Work out the finished part from the listing and answer in its coordinate system (mm). A direction names the side the tool comes from. Round coordinates to 2 decimals unless told otherwise and drop trailing zeros. Loops run counter-clockwise (first coordinate to the right, second up) from the corner with the lowest first, then second, coordinate; pieces in that order, holes last.
```python
from build123d import *

# Parameters (mm, degrees)
F0_W      = 76.2
F0_H      = 38.1
F1_DEPTH  = 25.4
F2_R      = 6.35
F1_FACE_W = 76.2
F1_FACE_H = 38.1
F3_DEPTH  = 25.4
F4_SIZE   = 2.53999
F5_R      = 10.16
F6_DEPTH  = 38.1
F7_R      = 5.08
F8_DEPTH  = 6.35
F9_R      = 10.16
F10_DEPTH = 6.35
F11_R     = 1.905
F12_DEPTH = 25.4
F13_DEPTH = 15.24
F14_R     = 2.54
F15_R     = 2.54
F16_R     = 2.54
F17_DEPTH = 50.8
F18_SIZE  = 3.81
F19_R     = 5.07999


# Not quite as in the source:
# - a fillet or chamfer is up to 0.001 mm smaller than in the source, because OpenCascade refuses the exact size


with BuildPart() as f1:
    # F0 (on Top) → F1 (new body)
    with BuildSketch(Plane.XY):
        with Locations((-5.318582058, 0.8709464072)):
            Rectangle(F0_W, F0_H)
    extrude(amount=F1_DEPTH)

    # F2 (on Top) + F1_face (on face) → F3 (cut)
    with BuildSketch(Plane.XY):
        with Locations((-34.528582058, -9.2890535928)):
            Circle(F2_R)
        with Locations((23.891417942, 11.0309464072)):
            Circle(F2_R)
        with Locations((23.891417942, -9.2890535928)):
            Circle(F2_R)
        with Locations((-34.528582058, 11.0309464072)):
            Circle(F2_R)
    with BuildSketch(Plane(origin=(-5.318582058, 0.8709464072, 25.4), x_dir=(1, 0, 0), z_dir=(0, 0, 1))):
        Rectangle(F1_FACE_W, F1_FACE_H)
    extrude(amount=F3_DEPTH, mode=Mode.SUBTRACT)

    # F4 (size 2.54 in the source; OpenCascade refuses exactly that, so slightly less here)
    f4_edges = [f1.edges().sort_by_distance(p)[0] for p in [
        (-5.318582, -18.179054, 25.4),
        (32.781418, 0.870946, 25.4),
        (-5.318582, 19.920946, 25.4),
        (-43.418582, 0.870946, 25.4),
    ]]
    chamfer(f4_edges, length=F4_SIZE)

    # F5 (on Top) → F6 (join)
    with BuildSketch(Plane.XY):
        with Locations((-5.3988754862, 0)):
            Circle(F5_R)
    extrude(amount=F6_DEPTH)

    # F7 (on face) → F8 (join)
    with BuildSketch(Plane.XY.offset(38.1)):
        with Locations((-5.3988754862, 0)):
            Circle(F7_R)
    extrude(amount=F8_DEPTH)

    # F9 (on face) → F10 (join)
    with BuildSketch(Plane.XY.offset(44.45)):
        with Locations((-5.3988754862, 0)):
            Circle(F9_R)
    extrude(amount=F10_DEPTH)

    # F11 (on Right) → F12 (join)
    with BuildSketch(Plane.YZ):
        with Locations((0, 40.6930105954)):
            Circle(F11_R)
    extrude(amount=-F12_DEPTH)

    # F11 (on Right) → F13 (join)
    with BuildSketch(Plane.YZ):
        with Locations((0, 40.6930105954)):
            Circle(F11_R)
    extrude(amount=F13_DEPTH)

    # F14
    f14_edges = [f1.edges().sort_by_distance(p)[0] for p in [
        (-15.558875, 0, 25.4),
    ]]
    fillet(f14_edges, radius=F14_R)

    # F15
    f15_edges = [f1.edges().sort_by_distance(p)[0] for p in [
        (-15.558875, 0, 50.8),
    ]]
    fillet(f15_edges, radius=F15_R)

    # F16 (on face) → F17 (cut)
    with BuildSketch(Plane.XY.offset(50.8)):
        with Locations((-5.3988754862, 0)):
            Circle(F16_R)
    extrude(amount=-F17_DEPTH, mode=Mode.SUBTRACT)

    # F18
    f18_edges = [f1.edges().sort_by_distance(p)[0] for p in [
        (32.781418, -18.179054, 11.430005),
        (-43.418582, -18.179054, 11.430005),
        (32.781418, 19.920946, 11.430005),
        (-43.418582, 19.920946, 11.430005),
    ]]
    chamfer(f18_edges, length=F18_SIZE)

    # F19 (radius 5.08 in the source; OpenCascade refuses exactly that, so slightly less here)
    f19_edges = [f1.edges().sort_by_distance(p)[0] for p in [
        (-15.558875, 0, 38.1),
    ]]
    fillet(f19_edges, radius=F19_R)


solid = f1.part
```
1. Determine the mould class of faces 4 (the face through (17.548, -9.01, 12.522)), 5 (the face through (32.781, 1, 11)), 6 (the face through (-6, 19.921, 11)) for opening direction Y: +Y half, -Y half, draft (parallel to the pull), parting line (faces both ways), or undercut.
Answer key:
face 4: undercut
face 5: draft
face 6: +Y half
2. Which of the six approach directions +Z, -Z, +X, -X, +Y, -Y give full straight-line access (tool end or side, diameter ignored) to faces 1 (the face through (-17.647, -0.413, 38.833)), 2 (the face through (15.24, 0, 41)), 3 (the face through (4.292, 3.052, 46.328))?
Answer key:
face 1: -X
face 2: +Z, +X, +Y, -Y
face 3: +Z
3. Given pin 1 (3 mm diameter, centred on x = -23.5, y = -13, fed in from -Z); pin 2 (6 mm diameter, centred on x = 20.5, y = -5.5, fed in from +Z); pin 3 (3 mm diameter, centred on y = -1, z = 40.5, fed in from +X); pin 4 (3 mm diameter, centred on y = 0.5, z = 40.5, fed in from -X), each flat-ended and moving along its own axis, determine where each tip first touches the part or whether it passes through.
Answer key:
pin 1: stops at z = 0
pin 2: stops at z = 25.4
pin 3: stops at x = 15.24
pin 4: stops at x = -25.4
4. Find section B-B (y = -13.5). Write down the section's boundary in (x, z), then the cut area to 3 significant figures.
Answer key:
outline: (-43.42, 0) - (-39.28, 0) - (-39.28, 25.4) - (-40.88, 25.4) - (-43.42, 22.86) - close; (-29.78, 0) - (19.14, 0) - (19.14, 25.4) - (-29.78, 25.4) - close; (28.64, 0) - (32.78, 0) - (32.78, 22.86) - (30.24, 25.4) - (28.64, 25.4) - close
area: 1,450 mm2
5. Consider probe 1 along Y at (x, z) = (24, 18); probe 2 along Y at (x, z) = (-34, 18); probe 3 along X at (y, z) = (-15, 7). Determine where each line is inside the solid, lowest interval first.
Answer key:
probe 1: y = -18.18 to -15.64, -2.94 to 4.68, 17.38 to 19.92
probe 2: y = -18.18 to -15.62, -2.96 to 4.7, 17.36 to 19.92
probe 3: x = -42.79 to -37.3, -31.75 to 21.12, 26.67 to 32.15
6. Find section A-A (x = -29.5). Write down the section's boundary in (y, z).
Answer key:
outline: (-18.18, 0) - (-13.17, 0) - (-13.17, 25.4) - (-15.64, 25.4) - (-18.18, 22.86) - close; (-5.41, 0) - (7.15, 0) - (7.15, 25.4) - (-5.41, 25.4) - close; (14.91, 0) - (19.92, 0) - (19.92, 22.86) - (17.38, 25.4) - (14.91, 25.4) - close
